Read the model definition and answer for the solid it produces. Units are mm, in the model's axes. A direction names the side the tool comes from. Coordinates: 2 decimals unless noted, no trailing zeros. Order: outer loops, then holes, each group sorted by start corner. A loop starts at its lowest first (then second) coordinate and runs counter-clockwise, first axis right, second up.
```python
from build123d import *

# Parameters (mm, degrees)
HOLE_WIZARD_M4_1_D           = 4.5
HOLE_WIZARD_M4_1_DEPTH       = 7
HOLE_WIZARD_M4_1_CSINK_D     = 9.4
HOLE_WIZARD_M4_1_CSINK_ANGLE = 90
SKETCH_4_R                   = 3.75
CUT_EXTRUDE_M4_DEPTH         = 3
HOLE_WIZARD_M4_1_2_D         = 3.3
HOLE_WIZARD_M4_1_2_DEPTH     = 4


with BuildPart() as part:
    # 스케치1 → 회전1 (revolve)
    with BuildSketch(Plane.XY):
        Polygon((0, 0), (-15, 0), (-15, 2), (-14, 2), (-14, 7), (0, 7), align=None)
    revolve(axis=Axis((0, 0, 0), (0, 1, 0)))

    # Hole Wizard M4 _ _ _ _1
    with Locations(Plane(origin=(0, 7, 0), x_dir=(1, 0, 0), z_dir=(0, 1, 0))):
        with Locations((-7.5, 0), (7.5, 0)):
            CounterSinkHole(HOLE_WIZARD_M4_1_D / 2, HOLE_WIZARD_M4_1_CSINK_D / 2, depth=HOLE_WIZARD_M4_1_DEPTH, counter_sink_angle=HOLE_WIZARD_M4_1_CSINK_ANGLE)

    # 스케치4 → M4 둥근 머리 나사용 카운터싱크 (cut)
    with BuildSketch(Plane.XZ):
        Circle(SKETCH_4_R)
    extrude(amount=-CUT_EXTRUDE_M4_DEPTH, mode=Mode.SUBTRACT)

    # Hole Wizard M4 _ _1 2
    with Locations(Plane(origin=(0, 3, 0), x_dir=(-1, 0, 0), z_dir=(0, -1, 0))):
        with Locations((0, 0)):
            Hole(HOLE_WIZARD_M4_1_2_D / 2, depth=HOLE_WIZARD_M4_1_2_DEPTH)


solid = part.part
```
1) Straight lines are drawn through the part: line 1 (Z direction, x = 0, y = 1.25); line 2 (Z direction, x = 0, y = 6); line 3 (X direction, y = 6.75, z = 1.75). For each, find the intervals that lie inside material, in ascending order.
A:
line 1: z = -15 to -3.75, 3.75 to 15
line 2: z = -14 to -1.65, 1.65 to 14
line 3: x = -13.89 to -11.59, -3.41 to 3.41, 11.59 to 13.89
2) Which of the six approach directions +Z, -Z, +X, -X, +Y, -Y give full straight-line access (tool end or side, diameter ignored) to faces 4 (the cylindrical face through (9.748, 2.243, -0.099)), 5 (the flat face through (1, 3, -2))?
A:
face 4: +Y, -Y
face 5: -Y
3) A cutting plane is placed at B-B, the plane z = 0. Determine the outline of the cut face in (x, y).
A:
outline: (-15, 0) - (-9.75, 0) - (-9.75, 4.55) - (-12.2, 7) - (-14, 7) - (-14, 2) - (-15, 2) - close; (-5.25, 0) - (-3.75, 0) - (-3.75, 3) - (-1.65, 3) - (-1.65, 7) - (-2.8, 7) - (-5.25, 4.55) - close; (1.65, 3) - (3.75, 3) - (3.75, 0) - (5.25, 0) - (5.25, 4.55) - (2.8, 7) - (1.65, 7) - close; (9.75, 0) - (15, 0) - (15, 2) - (14, 2) - (14, 7) - (12.2, 7) - (9.75, 4.55) - close
4) A cutting plane is placed at A-A, the plane x = 0. Determine the outline of the cut face in (y, z).
A:
outline: (0, -15) - (2, -15) - (2, -14) - (7, -14) - (7, -1.65) - (3, -1.65) - (3, -3.75) - (0, -3.75) - close; (0, 3.75) - (3, 3.75) - (3, 1.65) - (7, 1.65) - (7, 14) - (2, 14) - (2, 15) - (0, 15) - close
5) A flat-ended cylindrical pin translates along its axis: pin 1 Ø4 at (x, y) = (7.5, 6) entering from +Z. Find the tip coordinate at first contact, or state that the pin passes through.
A:
pin 1: stops at z = 12.87
6) Determine the mould class of faces 1 (the cylindrical face through (-12.932, 4.535, -5.362)), 2 (the flat face through (0, 7, -3)), 3 (the cylindrical face through (-1.216, 5.028, -1.115)) for opening direction X: pulls with the +X half, pulls with the -X half, needs draft (parallel to the pull), parting line crosses it, or undercut.
A:
face 1: parting line crosses it
face 2: needs draft
face 3: undercut
7) A cutting plane is placed at C-C, the plane y = 6. Determine the outline of the cut face in (x, z), and give its area (3 significant figures).
A:
outline: circle Ø28 at (0, 0); hole circle Ø7.4 at (-7.5, 0); hole circle Ø3.3 at (0, 0); hole circle Ø7.4 at (7.5, 0)
area: 521 mm2
8) A cutting plane is placed at D-D, the plane z = -7.5. Determine the outline of the cut face in (x, y).
A:
outline: (-12.99, 0) - (12.99, 0) - (12.99, 2) - (11.82, 2) - (11.82, 7) - (-11.82, 7) - (-11.82, 2) - (-12.99, 2) - close
